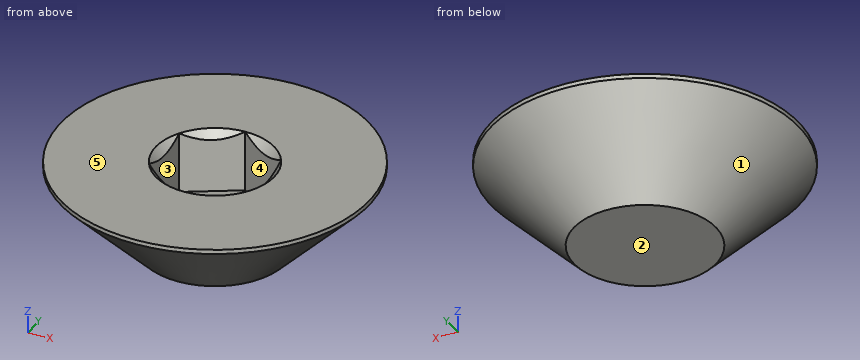
from build123d import *

# Parameters (mm, degrees)
CUT_EXTRUDE2_DEPTH = 1.19


with BuildPart() as part:
    # Sketch7 → Revolve2 (revolve)
    with BuildSketch(Plane(origin=(0, 0, 0), x_dir=(0, 0, -1), z_dir=(1, 0, 0)), mode=Mode.PRIVATE) as revolve2_sk:
        Polygon((-3, 3), (-2.915, 3), (-1.3, 1.385), (-1.3, 0), (-3, 0), align=None)
    revolve(revolve2_sk.sketch.rotate(Axis((0, 0, 3), (0, 0, -1)), 180), axis=Axis((0, 0, 3), (0, 0, -1)))

    # Sketch5 → Cut-Extrude2 (cut)
    with BuildSketch(Plane.XY.offset(3)):
        Polygon((1, -0.577350269), (1, 0.577350269), (0, 1.154700538), (-1, 0.577350269), (-1, -0.577350269), (0, -1.154700538), align=None)
    extrude(amount=-CUT_EXTRUDE2_DEPTH, mode=Mode.SUBTRACT)

    # Cut-Extrude3 cone 1 section (through the dimple's axis) → Cut-Extrude3 (revolve, cut)
    with BuildSketch(Plane(origin=(0, 0, 3), x_dir=(0, -1, 0), z_dir=(1, 0, 0))):
        Polygon((0, 0), (1.154700538, 0), (0, 1.154700538), align=None)
    revolve(axis=Axis((0, 0, 3), (0, 0, -1)), mode=Mode.SUBTRACT)


solid = part.part
Verification items for the finished model (mm, model axes). Face numbers are marked on the shaded views. A direction names the side the tool comes from. Give positions to 0.01 mm unless a question says otherwise; leave off trailing zeros. Order: outer loops, then holes, each group sorted by start corner. A loop starts at its lowest first (then second) coordinate and runs counter-clockwise, first axis right, second up. Notation, with made-up numbers: M -37.5,41.25 L -19.5,41.25 A19 ccw -19.5,52.25 Z; hole C -23.5,22.25 d7. An arc over 180 degrees is marked long. Use one line per item in the form item = value. Start each with the question number.
Q1. Section check B-B (z = 2.45). Enter the section's corners in (x, y) (3 decimals).
Q2. Scan lines: line 1 along Y through (x, z) = (0.55, 2.55); line 2 along X through (y, z) = (-0.15, 2.3); line 3 along X through (y, z) = (-0.35, 2.45). Record each from-to range of solid material in increasing order. Write a range as [from, to].
Q3. Section check D-D (z = 1.6). Enter the section's corners in (x, y) (3 decimals).
Q4. Access from +Z, -Z, +X, -X, +Y, -Y to the whole of each face (thin tool, end or side, straight path). Record for the marked faces 4 and 5.
Q5. Section check A-A (y = 0). Enter the section's corners in (x, z) (3 decimals), then the cut area to 3 significant figures.
Q6. Mould release check, pull along Y, two halves, no side actions. Record for the marked faces 1, 2 and 3: +Y half, -Y half, draft (parallel to the pull), parting line (faces both ways), or undercut.
Q7. Section check C-C (z = 2.1). Enter the section's corners in (x, y) (3 decimals).
Evaluation:
q1.outline = C 0,0 d5.07; hole M -1,-0.577 L 0,-1.155 L 1,-0.577 L 1,0.577 L 0,1.155 L -1,0.577 Z
q2.line_1 = [-2.58, -0.84], [0.84, 2.58]
q2.line_2 = [-2.38, -1], [1, 2.38]
q2.line_3 = [-2.51, -1], [1, 2.51]
q3.outline = C 0,0 d3.37
q4.face_4 = +Z
q4.face_5 = +Z, +X, -X, +Y, -Y
q5.outline = M -3,2.915 L -1.385,1.3 L 1.385,1.3 L 3,2.915 L 3,3 L 1.155,3 L 1,2.845 L 1,1.81 L -1,1.81 L -1,2.845 L -1.155,3 L -3,3 Z
q5.area = 5.19 mm2
q6.face_1 = parting line
q6.face_2 = draft
q6.face_3 = undercut
q7.outline = C 0,0 d4.37; hole M -1,-0.577 L 0,-1.155 L 1,-0.577 L 1,0.577 L 0,1.155 L -1,0.577 Z
